from build123d import *

# Parameters (mm, degrees)
F0_W     = 23.412162
F0_H     = 100
F1_DEPTH = 25
F2_W     = 14.901995
F2_H     = 20
F3_DEPTH = 40


with BuildPart() as f1:
    # F0 (on Front) → F1 (new body)
    with BuildSketch(Plane.XZ):
        with Locations((11.706081, 50)):
            Rectangle(F0_W, F0_H)
    extrude(amount=F1_DEPTH)

    # F2 (on face) → F3 (join)
    with BuildSketch(Plane.YZ.offset(23.412162)):
        with Locations((-17.549003, 60)):
            Rectangle(F2_W, F2_H)
        with Locations((-17.549003, 40)):
            Rectangle(F2_W, F2_H)
    extrude(amount=F3_DEPTH)


solid = f1.part
Could you check a few things on this model? Use its own coordinates, in mm. A direction names the side the tool comes from. Give positions to 0.01 mm unless a question says otherwise; leave off trailing zeros. Write each loop counter-clockwise with the first axis right and the second up, starting at its lowest first coordinate (ties: lowest second). Pieces come first, ordered by that corner, then holes. Notation, with made-up numbers: (-24, 7.25) -> (1, 7.25) arc R25 ccw to (1, 25.25) -> close; hole circle Ø1 at (20.25, 61.5). An arc over 180 degrees is marked (long way). Write each question's results on one line, items separated by ' | '. Start each with the question number.
Q1. I need wall thicknesses on probe 1 along X at (y, z) = (-10.5, 10); probe 2 along Z at (x, y) = (51, -22.25); probe 3 along Y at (x, z) = (46, 42). Which ranges of each line are inside material? Lowest first, please.
Q2. Suppose I cut it at A-A, the plane y = -23. List the corners of the cut face in (x, z) for me.
Q3. Which directions (+Z, -Z, +X, -X, +Y, -Y) give clear straight access to the entire face, cutting with the end or side of a thin tool? Please do faces 1 (the face through (12, -12, 100)), 2 (the face through (63.412, -18, 50)), 3 (the face through (43, -10.098, 50)), 4 (the face through (43, -18, 30)), 5 (the face through (43, -18, 70)).
Q4. Suppose I cut it at D-D, the plane z = 63. List the corners of the cut face in (x, y) for me, and give its area (3 significant figures).
Q5. I'm going to push flat-ended pins straight in: pin 1 Ø4.5 at (x, y) = (34.5, -16.5) entering from -Z; pin 2 Ø10 at (x, z) = (44.5, 41.5) entering from +Y; pin 3 Ø7.5 at (y, z) = (-8.5, 42.5) entering from +X; pin 4 Ø8 at (x, y) = (53, -16) entering from +Z. Where does each tip first touch, or does it pass through?
Q6. Suppose I cut it at B-B, the plane z = 74.5. List the corners of the cut face in (x, y) for me, and give its area (3 significant figures).
Q7. Suppose I cut it at C-C, the plane x = 47. List the corners of the cut face in (y, z) for me.
Outcome:
1) probe 1: 0 to 23.41 | probe 2: 30 to 70 | probe 3: -25 to -10.1
2) outline: (0, 0) -> (23.41, 0) -> (23.41, 30) -> (63.41, 30) -> (63.41, 70) -> (23.41, 70) -> (23.41, 100) -> (0, 100) -> close
3) face 1: +Z, +X, -X, +Y, -Y | face 2: +Z, -Z, +X, +Y, -Y | face 3: +Z, -Z, +X, +Y | face 4: -Z, +X, +Y, -Y | face 5: +Z, +X, +Y, -Y
4) outline: (0, -25) -> (63.41, -25) -> (63.41, -10.1) -> (23.41, -10.1) -> (23.41, 0) -> (0, 0) -> close | area: 1,180 mm2
5) pin 1: z = 30 | pin 2: y = -10.1 | pin 3: x = 63.41 | pin 4: z = 70
6) outline: (0, -25) -> (23.41, -25) -> (23.41, 0) -> (0, 0) -> close | area: 585 mm2
7) outline: (-25, 30) -> (-10.1, 30) -> (-10.1, 70) -> (-25, 70) -> close
